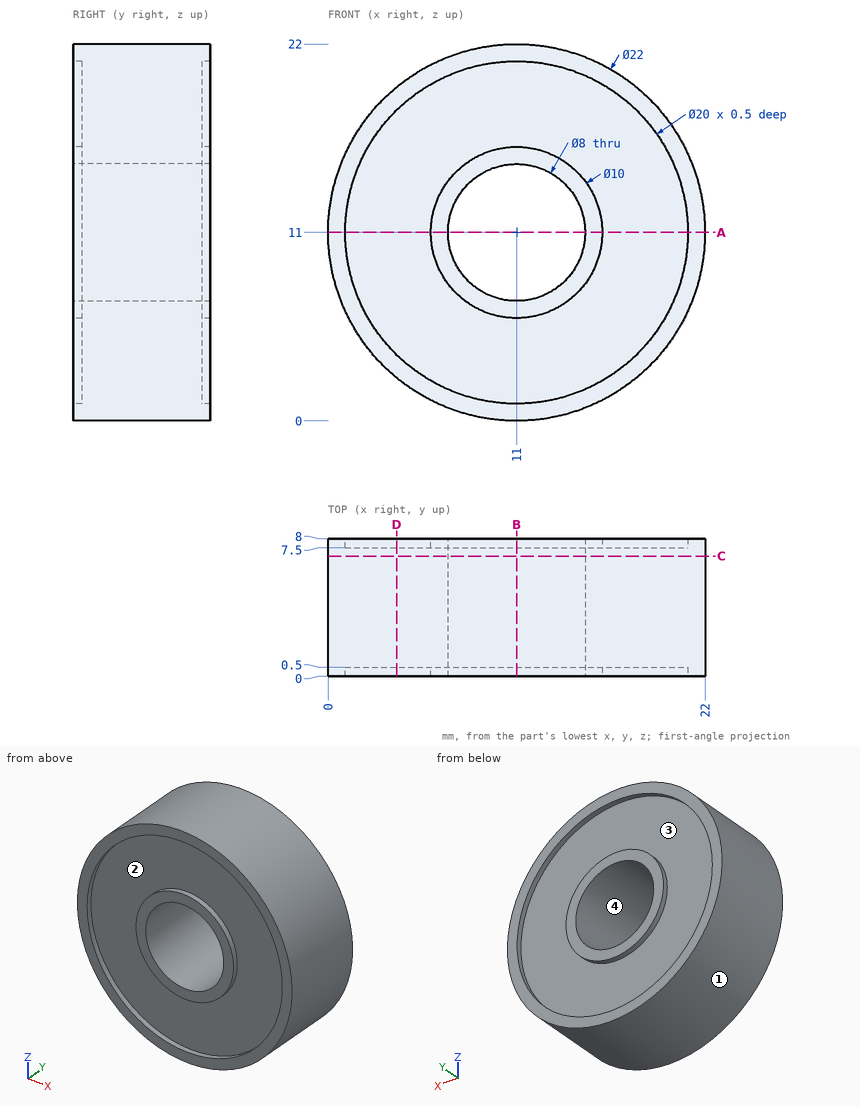
Input: dimensioned drawing with shaded views. Units: mm. Origin: part minimum x, y, z. A direction names the side the tool comes from. Coordinates: 2 decimals unless noted, no trailing zeros. Order: outer loops, then holes, each group sorted by start corner. A loop starts at its lowest first (then second) coordinate and runs counter-clockwise, first axis right, second up. Notation, with made-up numbers: (73.5, 48.5) - (89.5, 48.5) arc R23 ccw to (89.5, 58.5) - close; hole circle Ø2 at (-9.75, 54.5). An arc over 180 degrees is marked (long way). Put each result on its own line as item: value.
1. Cut plane C-C on y = 7. Return the cut outline in (x, z), then the cut area to 3 significant figures.
Report:
outline: circle Ø22 at (11, 11); hole circle Ø8 at (11, 11)
area: 330 mm2
2. Contact query for flat-ended pins moving along their axis: pin 1 Ø2 at (x, z) = (7.5, 5) entering from -Y; pin 2 Ø4 at (y, z) = (1.5, 13.5) entering from +X; pin 3 Ø2 at (x, z) = (9, 12.5) entering from +Y. Output: stop coordinate, or through.
Report:
pin 1: stops at y = 0.5
pin 2: stops at x = 21.99
pin 3: passes through
3. Line query: line 1 along Z through (x, y) = (11, 7.75); line 2 along Z through (x, y) = (11, 2); line 3 along X through (y, z) = (7.75, 12.5). Output: solid intervals per line, ascending.
Report:
line 1: z = 0 to 1, 6 to 7, 15 to 16, 21 to 22
line 2: z = 0 to 7, 15 to 22
line 3: x = 0.1 to 1.11, 6.23 to 7.29, 14.71 to 15.77, 20.89 to 21.9
4. Cut plane D-D on x = 4. Return the cut outline in (y, z), then the cut area to 3 significant figures.
Report:
outline: (0, 2.51) - (8, 2.51) - (8, 3.86) - (7.5, 3.86) - (7.5, 18.14) - (8, 18.14) - (8, 19.49) - (0, 19.49) - (0, 18.14) - (0.5, 18.14) - (0.5, 3.86) - (0, 3.86) - close
area: 121 mm2
5. Reachability of the marked faces 3 and 4 from +Z, -Z, +X, -X, +Y, -Y: full face, straight path, thin tool, end or side. Return the list, or none.
Report:
face 3: +Y
face 4: +Y, -Y
6. Cut plane A-A on z = 11. Return the cut outline in (x, y), then the cut area to 3 significant figures.
Report:
outline: (0, 0) - (1, 0) - (1, 0.5) - (6, 0.5) - (6, 0) - (7, 0) - (7, 8) - (6, 8) - (6, 7.5) - (1, 7.5) - (1, 8) - (0, 8) - close; (15, 0) - (16, 0) - (16, 0.5) - (21, 0.5) - (21, 0) - (22, 0) - (22, 8) - (21, 8) - (21, 7.5) - (16, 7.5) - (16, 8) - (15, 8) - close
area: 102 mm2
7. Cut plane B-B on x = 11. Return the cut outline in (y, z), then the cut area to 3 significant figures.
Report:
outline: (0, 0) - (8, 0) - (8, 1) - (7.5, 1) - (7.5, 6) - (8, 6) - (8, 7) - (0, 7) - (0, 6) - (0.5, 6) - (0.5, 1) - (0, 1) - close; (0, 15) - (8, 15) - (8, 16) - (7.5, 16) - (7.5, 21) - (8, 21) - (8, 22) - (0, 22) - (0, 21) - (0.5, 21) - (0.5, 16) - (0, 16) - close
area: 102 mm2
8. Draft query along X for the marked faces 1 and 2. Return one class per face: pulls with the +X half, pulls with the -X half, needs draft (parallel to the pull), parting line crosses it, or undercut.
Report:
face 1: parting line crosses it
face 2: undercut
